Read the model definition and answer for the solid it produces. Units are mm, in the model's axes. Coordinates: 2 decimals unless noted, no trailing zeros. Write item = value, one per line. Start each with the question number.
1) Find the intervals of material crossed by line 1 along Y through (x, z) = (148, 0.9), in increasing order. Write a range as from..to.
2) Section A-A (y = 6.25) is taken. Count the separate pieces of the cut face and the enclosed holes in it, plus the area to 3 significant figures.
3) A flat-ended cylindrical pin translates along its axis: pin 1 Ø0.6 at (x, z) = (215, -0.5) entering from +Y. Find the tip coordinate at first contact, or state that the pin passes through.
from build123d import *

# Parameters (mm, degrees)
ESQUISSE1_W                = 500
ESQUISSE1_H                = 20
BOSS_EXTRU_1_DEPTH         = 1
ESQUISSE2_W                = 2
ESQUISSE2_H                = 10
ENL_V_MAT_EXTRU_1_DEPTH    = 3
R_P_TITION_LIN_AIRE1_COUNT = 7
R_P_TITION_LIN_AIRE1_PITCH = 33
SYM_TRIE1_COPY_1_SKETCH_W  = 2
SYM_TRIE1_COPY_1_SKETCH_H  = 10
SYM_TRIE1_COPY_1_DEPTH     = 3
SYM_TRIE1_COPY_2_SKETCH_W  = 2
SYM_TRIE1_COPY_2_SKETCH_H  = 10
SYM_TRIE1_COPY_2_DEPTH     = 3
SYM_TRIE1_COPY_3_SKETCH_W  = 2
SYM_TRIE1_COPY_3_SKETCH_H  = 10
SYM_TRIE1_COPY_3_DEPTH     = 3
SYM_TRIE1_COPY_4_SKETCH_W  = 2
SYM_TRIE1_COPY_4_SKETCH_H  = 10
SYM_TRIE1_COPY_4_DEPTH     = 3
SYM_TRIE1_COPY_5_SKETCH_W  = 2
SYM_TRIE1_COPY_5_SKETCH_H  = 10
SYM_TRIE1_COPY_5_DEPTH     = 3
SYM_TRIE1_COPY_6_SKETCH_W  = 2
SYM_TRIE1_COPY_6_SKETCH_H  = 10
SYM_TRIE1_COPY_6_DEPTH     = 3


with BuildPart() as part:
    # Esquisse1 → Boss.-Extru.1 (new body, symmetric)
    with BuildSketch(Plane.XY):
        Rectangle(ESQUISSE1_W, ESQUISSE1_H)
    extrude(amount=BOSS_EXTRU_1_DEPTH, both=True)

    # Esquisse2 → Enlèv. mat.-Extru.1 (cut, through all)
    with BuildSketch(Plane.XY.offset(1)):
        with Locations((16.5, 5)):
            Rectangle(ESQUISSE2_W, ESQUISSE2_H)
    enl_v_mat_extru_1 = extrude(amount=-ENL_V_MAT_EXTRU_1_DEPTH, mode=Mode.SUBTRACT)

    # Répétition linéaire1: Enlèv. mat.-Extru.1 ×7
    with Locations(*[(i * R_P_TITION_LIN_AIRE1_PITCH, 0, 0) for i in range(1, R_P_TITION_LIN_AIRE1_COUNT)]):
        add(enl_v_mat_extru_1, mode=Mode.SUBTRACT)

    # Symétrie1: Enlèv. mat.-Extru.1 across plane
    add(enl_v_mat_extru_1.mirror(Plane(origin=(0, 0, 0), x_dir=(0, 0, 1), z_dir=(1, 0, 0))), mode=Mode.SUBTRACT)

    # Symétrie1 copy 1 sketch → Symétrie1 copy 1 (cut, through all)
    with BuildSketch(Plane(origin=(-33, 0, 1), x_dir=(-1, 0, 0), z_dir=(0, 0, 1))):
        with Locations((16.5, -5)):
            Rectangle(SYM_TRIE1_COPY_1_SKETCH_W, SYM_TRIE1_COPY_1_SKETCH_H)
    extrude(amount=-SYM_TRIE1_COPY_1_DEPTH, mode=Mode.SUBTRACT)

    # Symétrie1 copy 2 sketch → Symétrie1 copy 2 (cut, through all)
    with BuildSketch(Plane(origin=(-66, 0, 1), x_dir=(-1, 0, 0), z_dir=(0, 0, 1))):
        with Locations((16.5, -5)):
            Rectangle(SYM_TRIE1_COPY_2_SKETCH_W, SYM_TRIE1_COPY_2_SKETCH_H)
    extrude(amount=-SYM_TRIE1_COPY_2_DEPTH, mode=Mode.SUBTRACT)

    # Symétrie1 copy 3 sketch → Symétrie1 copy 3 (cut, through all)
    with BuildSketch(Plane(origin=(-99, 0, 1), x_dir=(-1, 0, 0), z_dir=(0, 0, 1))):
        with Locations((16.5, -5)):
            Rectangle(SYM_TRIE1_COPY_3_SKETCH_W, SYM_TRIE1_COPY_3_SKETCH_H)
    extrude(amount=-SYM_TRIE1_COPY_3_DEPTH, mode=Mode.SUBTRACT)

    # Symétrie1 copy 4 sketch → Symétrie1 copy 4 (cut, through all)
    with BuildSketch(Plane(origin=(-132, 0, 1), x_dir=(-1, 0, 0), z_dir=(0, 0, 1))):
        with Locations((16.5, -5)):
            Rectangle(SYM_TRIE1_COPY_4_SKETCH_W, SYM_TRIE1_COPY_4_SKETCH_H)
    extrude(amount=-SYM_TRIE1_COPY_4_DEPTH, mode=Mode.SUBTRACT)

    # Symétrie1 copy 5 sketch → Symétrie1 copy 5 (cut, through all)
    with BuildSketch(Plane(origin=(-165, 0, 1), x_dir=(-1, 0, 0), z_dir=(0, 0, 1))):
        with Locations((16.5, -5)):
            Rectangle(SYM_TRIE1_COPY_5_SKETCH_W, SYM_TRIE1_COPY_5_SKETCH_H)
    extrude(amount=-SYM_TRIE1_COPY_5_DEPTH, mode=Mode.SUBTRACT)

    # Symétrie1 copy 6 sketch → Symétrie1 copy 6 (cut, through all)
    with BuildSketch(Plane(origin=(-198, 0, 1), x_dir=(-1, 0, 0), z_dir=(0, 0, 1))):
        with Locations((16.5, -5)):
            Rectangle(SYM_TRIE1_COPY_6_SKETCH_W, SYM_TRIE1_COPY_6_SKETCH_H)
    extrude(amount=-SYM_TRIE1_COPY_6_DEPTH, mode=Mode.SUBTRACT)


solid = part.part
Answer key:
q1.line_1 = -10..0
q2.separate_pieces = 15
q2.enclosed_holes = 0
q2.area = 944 mm^2
q3.pin_1 = 0
